Could you check a few things on this drawing? It's one solid part, dimensions in mm from its lowest x, y, z. A direction names the side the tool comes from. Coordinates: 2 decimals unless noted, no trailing zeros. Write each loop counter-clockwise with the first axis right and the second up, starting at its lowest first coordinate (ties: lowest second). Pieces come first, ordered by that corner, then holes. Notation, with made-up numbers: M -16.5,43.25 L -10.5,43.25 A32 ccw -10.5,82.25 Z; hole C 45.5,-10 d3. An arc over 180 degrees is marked long. Use a Markdown table: item, result.
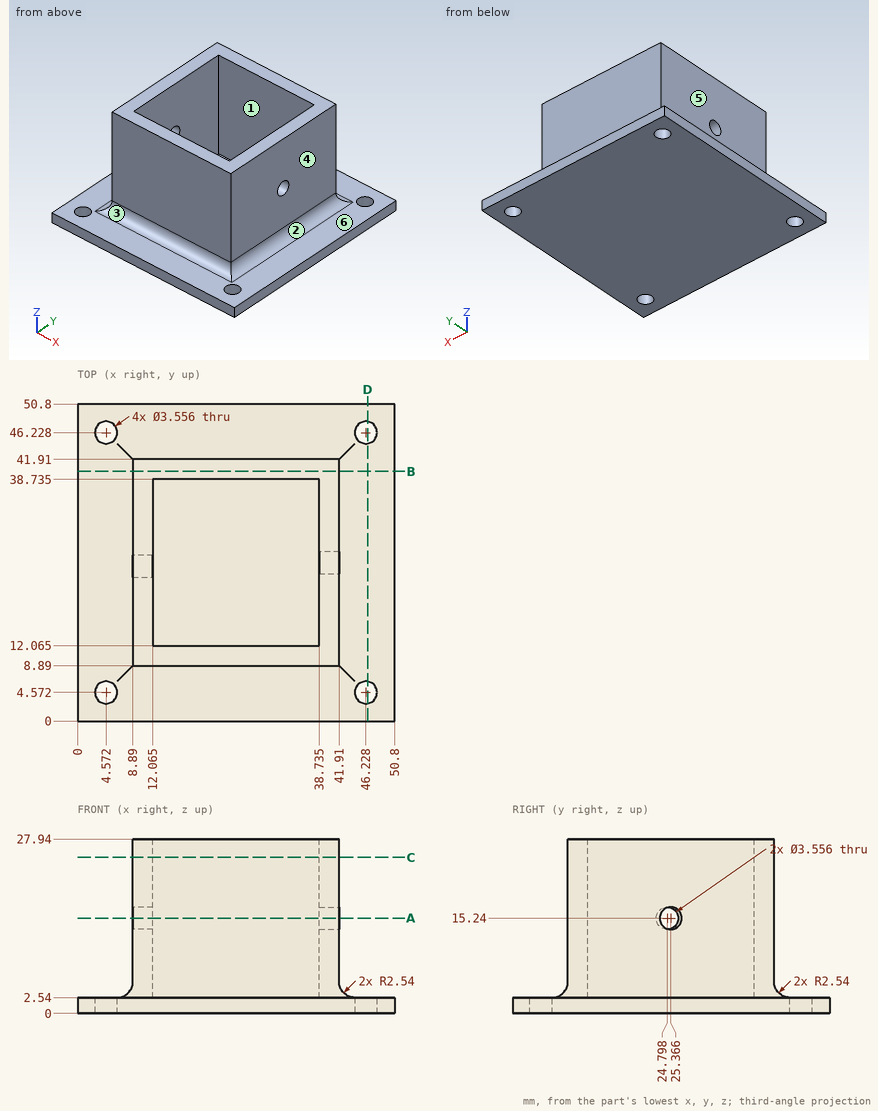
1. Suppose I cut it at B-B on y = 40. Write out the boundary of the cut face in (x, z).
Answers follow:
| item | result |
|---|---|
| outline | M 0,0 L 50.8,0 L 50.8,2.54 L 44.45,2.54 A2.54 cw 41.91,5.08 L 41.91,27.94 L 8.89,27.94 L 8.89,5.08 A2.54 cw 6.35,2.54 L 0,2.54 Z |
2. We'd pull the mould along Y, two halves only. Please class the marked faces 1, 2 and 3: +Y half, -Y half, draft (parallel to the pull), parting line (faces both ways), or undercut.
Answers follow:
| item | result |
|---|---|
| face 1 | undercut |
| face 2 | draft |
| face 3 | -Y half |
3. I need wall thicknesses on probe 1 along Y at (x, z) = (17, 18) (1 decimal); probe 2 along Z at (x, y) = (5, 22). Which ranges of each line are inside material? Lowest first, please.
Answers follow:
| item | result |
|---|---|
| probe 1 | y = 8.9 to 12.1, 38.7 to 41.9 |
| probe 2 | z = 0 to 2.54 |
4. Suppose I cut it at A-A on z = 15.24. Write out the boundary of the cut face in (x, y) (1 decimal).
Answers follow:
| item | result |
|---|---|
| outline | M 8.9,8.9 L 41.9,8.9 L 41.9,23.6 L 38.7,23.6 L 38.7,12.1 L 12.1,12.1 L 12.1,23 L 8.9,23 Z; M 8.9,26.6 L 12.1,26.6 L 12.1,38.7 L 38.7,38.7 L 38.7,27.1 L 41.9,27.1 L 41.9,41.9 L 8.9,41.9 Z |
5. Suppose I cut it at D-D on x = 46.5. Write out the boundary of the cut face in (y, z) (1 decimal).
Answers follow:
| item | result |
|---|---|
| outline | M 0,0 L 2.8,0 L 2.8,2.5 L 0,2.5 Z; M 6.3,0 L 44.5,0 L 44.5,2.5 L 6.3,2.5 Z; M 48,0 L 50.8,0 L 50.8,2.5 L 48,2.5 Z |
6. Suppose I cut it at C-C on z = 25. Write out the boundary of the cut face in (x, y) (1 decimal), and give its area (3 significant figures).
Answers follow:
| item | result |
|---|---|
| outline | M 8.9,8.9 L 41.9,8.9 L 41.9,41.9 L 8.9,41.9 Z; hole M 12.1,12.1 L 38.7,12.1 L 38.7,38.7 L 12.1,38.7 Z |
| area | 379 mm2 |
7. Will these pins go through, and if not, where does the flat tip stop? pin 1 Ø6 at (x, z) = (38, 8) entering from +Y; pin 2 Ø5 at (x, z) = (36, 13.5) entering from -Y; pin 3 Ø8 at (x, y) = (27, 28) entering from +Z.
Answers follow:
| item | result |
|---|---|
| pin 1 | stops at y = 41.91 |
| pin 2 | stops at y = 8.89 |
| pin 3 | stops at z = 2.54 |
8. Which directions (+Z, -Z, +X, -X, +Y, -Y) give clear straight access to the entire face, cutting with the end or side of a thin tool? Please do the marked faces 4, 5 and 6.
Answers follow:
| item | result |
|---|---|
| face 4 | +Z, +X, +Y, -Y |
| face 5 | +Z, -X, +Y, -Y |
| face 6 | +Z |
